Work out the finished part from the listing and answer in its coordinate system (mm). A direction names the side the tool comes from. Round coordinates to 2 decimals unless told otherwise and drop trailing zeros. Loops run counter-clockwise (first coordinate to the right, second up) from the corner with the lowest first, then second, coordinate; pieces in that order, holes last.
```python
from build123d import *

# Parameters (mm, degrees)
F0_W         = 279.4
F0_H         = 482.6
F1_DEPTH     = 25.4
F2_R         = 5.08
F3_R         = 5.08
F4_W         = 176.9686788321
F4_H         = 19.3408131599
F5_DEPTH     = 25.4
F6_W         = 167.2982573509
F6_H         = 19.3408429623
F7_DEPTH     = 25.4
F8_W         = 152.4
F8_H         = 152.4
F9_DEPTH     = 25.4
F10_T        = 2.54
F10_T3_DEPTH = 157.48
F10_T5_DEPTH = 157.48
F10_T7_DEPTH = 30.48
F11_W        = 39.6487191319
F11_H        = 63.5
F12_DEPTH    = 25.4
F13_R        = 7.7119354401
F14_DEPTH    = 50.8


# Not quite as in the source:
# - a shell that OpenCascade refuses in one call is made with other operations: the cavity is built on its own and cut out


with BuildPart() as f1:
    # F0 (on Right) → F1 (new body)
    with BuildSketch(Plane.YZ):
        Rectangle(F0_W, F0_H)
    extrude(amount=F1_DEPTH)

    # F2
    f2_edges = [f1.edges().sort_by_distance(p)[0] for p in [
        (0, 139.7, 0),
        (0, 0, 241.3),
        (0, -139.7, 0),
        (0, 0, -241.3),
    ]]
    fillet(f2_edges, radius=F2_R)

    # F3
    f3_edges = [f1.edges().sort_by_distance(p)[0] for p in [
        (25.4, 139.7, 0),
        (25.4, 0, 241.3),
        (25.4, -139.7, 0),
        (25.4, 0, -241.3),
    ]]
    fillet(f3_edges, radius=F3_R)

    # F4 (on face) → F5 (cut)
    with BuildSketch(Plane(origin=(0, 0, 0), x_dir=(0, -1, 0), z_dir=(-1, 0, 0))):
        with Locations((0, 155.2102416754)):
            Rectangle(F4_W, F4_H)
    extrude(amount=-F5_DEPTH, mode=Mode.SUBTRACT)

    # F6 (on face) → F7 (cut)
    with BuildSketch(Plane.YZ.offset(25.4)):
        with Locations((0, 109.7592636943)):
            Rectangle(F6_W, F6_H)
    extrude(amount=-F7_DEPTH, mode=Mode.SUBTRACT)

    # F8 (on face) → F9 (join)
    with BuildSketch(Plane(origin=(0, 0, 0), x_dir=(0, -1, 0), z_dir=(-1, 0, 0))):
        Rectangle(F8_W, F8_H)
    extrude(amount=F9_DEPTH)

    # F10: shell of thickness 2.54, made by hand


with BuildPart() as f10_core1:
    # F10_t2: copy of F1
    add(f1.part)

    # the walls: a layer under each face that stays
    f10_faces = [f10_core1.faces().sort_by_distance(p)[0] for p in [
        (12.7, 139.7, 0),
        (12.7, 0, -241.3),
        (23.912103095, 138.2121018019, 0),
        (1.4878975516, 138.2121024484, 0),
        (12.7, 0, 241.3),
        (12.7, -139.7, 0),
        (23.912103095, 0, -239.8121018019),
        (1.4878975516, 0, -239.8121024484),
        (25.4, 0, 0),
        (23.912103095, 0, 239.8121018019),
        (0, -89.7466666667, -157.48),
        (1.4878975516, 0, 239.8121024484),
        (23.912103095, -138.2121018019, 0),
        (1.4878975516, -138.2121024484, 0),
        (12.7, 0, 119.4296851754),
        (12.7, -83.6491286755, 109.7592636943),
        (12.7, 0, 100.0888422132),
        (12.7, 83.6491286755, 109.7592636943),
        (12.7, -88.484339416, 155.2102416754),
        (12.7, 0, 145.5398350954),
        (12.7, 0, 164.8806482553),
        (12.7, 88.484339416, 155.2102416754),
        (-12.7, -76.2, 0),
        (-12.7, 0, -76.2),
        (-12.7, 76.2, 0),
        (-12.7, 0, 76.2),
    ]]
    thicken(f10_faces, amount=-F10_T, mode=Mode.SUBTRACT)

    # F10_s4 → F10_t3 (cut)
    with BuildSketch(Plane.XY.offset(-78.74)):
        Polygon((-0.0254, -76.2254), (2.54, -76.2), (2.54, -73.66), (0, -73.66), align=None)
        Polygon((-0.0254, 76.2254), (2.54, 76.2), (2.54, 73.66), (0, 73.66), align=None)
    extrude(amount=F10_T3_DEPTH, mode=Mode.SUBTRACT)

    # F10_s6 → F10_t5 (cut)
    with BuildSketch(Plane.XZ.offset(-78.74)):
        Polygon((-0.0254, -76.2254), (2.54, -76.2), (2.54, -73.66), (0, -73.66), align=None)
        Polygon((-0.0254, 76.2254), (2.54, 76.2), (2.54, 73.66), (0, 73.66), align=None)
    extrude(amount=F10_T5_DEPTH, mode=Mode.SUBTRACT)

    # F10_s8 → F10_t7 (cut)
    with BuildSketch(Plane.YZ.offset(-2.54)):
        Polygon((83.6237286755, 119.4042851754), (83.6491286755, 121.9696851754), (86.1891286755, 121.9696851754), (86.1891286755, 119.4296851754), align=None)
        Polygon((-83.6237286755, 119.4042851754), (-83.6491286755, 121.9696851754), (-86.1891286755, 121.9696851754), (-86.1891286755, 119.4296851754), align=None)
        Polygon((-83.6237286755, 100.1142422132), (-86.1891286755, 100.0888422132), (-86.1891286755, 97.5488422132), (-83.6491286755, 97.5488422132), align=None)
        Polygon((83.6237286755, 100.1142422132), (83.6491286755, 97.5488422132), (86.1891286755, 97.5488422132), (86.1891286755, 100.0888422132), align=None)
        Polygon((-88.458939416, 145.5652350954), (-91.024339416, 145.5398350954), (-91.024339416, 142.9998350954), (-88.484339416, 142.9998350954), align=None)
        Polygon((-88.458939416, 164.8552482553), (-91.024339416, 164.8806482553), (-91.024339416, 167.4206482553), (-88.484339416, 167.4206482553), align=None)
        Polygon((88.458939416, 145.5652350954), (88.484339416, 142.9998350954), (91.024339416, 142.9998350954), (91.024339416, 145.5398350954), align=None)
        Polygon((88.458939416, 164.8552482553), (88.484339416, 167.4206482553), (91.024339416, 167.4206482553), (91.024339416, 164.8806482553), align=None)
    extrude(amount=F10_T7_DEPTH, mode=Mode.SUBTRACT)


with BuildPart() as f1_1:
    add(f1.part)

    # what is left inside the walls is the cavity
    f10_cavity = [f10_core1.part.solids().sort_by_distance(p)[0] for p in [
        (22.8346, 0, -78.74),
    ]]
    add(f10_cavity, mode=Mode.SUBTRACT)

    # F11 (on face) → F12 (join)
    with BuildSketch(Plane(origin=(0, 0, 0), x_dir=(0, -1, 0), z_dir=(-1, 0, 0))):
        with Locations((0, 44.45)):
            Rectangle(F11_W, F11_H)
    extrude(amount=F12_DEPTH)

    # F13 (on face) → F14 (cut)
    with BuildSketch(Plane(origin=(0, 19.824359566, 0), x_dir=(-1, 0, 0), z_dir=(0, 1, 0))):
        with Locations((12.3025374487, 43.18)):
            Circle(F13_R)
    extrude(amount=-F14_DEPTH, mode=Mode.SUBTRACT)


solid = f1_1.part
```
1. Find section D-D (z = -185.5). Write down the section's boundary in (x, y), then the cut area to 3 significant figures.
Answer key:
outline: (0, -134.62) arc R5.08 ccw to (5.08, -139.7) - (20.32, -139.7) arc R5.08 ccw to (25.4, -134.62) - (25.4, 134.62) arc R5.08 ccw to (20.32, 139.7) - (5.08, 139.7) arc R5.08 ccw to (0, 134.62) - close; hole (2.54, -134.62) arc R2.54 ccw to (5.08, -137.16) - (20.32, -137.16) arc R2.54 ccw to (22.86, -134.62) - (22.86, 134.62) arc R2.54 ccw to (20.32, 137.16) - (5.08, 137.16) arc R2.54 ccw to (2.54, 134.62) - close
area: 1,510 mm2
2. Consider probe 1 along X at (y, z) = (9, 43); probe 2 along Z at (x, y) = (13, -1.5); probe 3 along Y at (x, z) = (-9, 37). Determine where each line is inside the solid, lowest interval first.
Answer key:
probe 1: x = -25.4 to -20.01, -4.59 to 0, 22.86 to 25.4
probe 2: z = -241.3 to -238.76, 97.55 to 100.09, 119.43 to 121.97, 143 to 145.54, 164.88 to 167.42, 238.76 to 241.3
probe 3: y = -76.2 to -73.66, 73.66 to 76.2
3. Find section C-C (z = 43.18). Give the number of separate pieces and of enclosed holes in the cut face, then the cut area to 3 significant figures.
Answer key:
separate pieces: 3
enclosed holes: 0
area: 1,660 mm2
4. Given pin 1 (3 mm diameter, centred on x = 0.5, z = -131.5, fed in from +Y); pin 2 (10 mm diameter, centred on x = -9.5, y = -18.5, fed in from +Z); pin 3 (4 mm diameter, centred on x = -19, z = 13.5, fed in from -Y), each flat-ended and moving along its own axis, determine where each tip first touches the part or whether it passes through.
Answer key:
pin 1: stops at y = 138.66
pin 2: stops at z = 76.2
pin 3: stops at y = -76.2
5. Which of the six approach directions +Z, -Z, +X, -X, +Y, -Y give full straight-line access (tool end or side, diameter ignored) to faces 4 (the face through (-21, -19.824, 43)), 5 (the face through (13, 1, 164.881)), 6 (the face through (13, 139.7, -3)), 7 (the face through (13, -1, 167.421)), 8 (the face through (25.4, -2, 3))?
Answer key:
face 4: -X
face 5: +X, -X
face 6: +Z, -Z, +X, -X, +Y
face 7: none
face 8: +Z, -Z, +X, +Y, -Y
6. Find section B-B (y = -104.5). Write down the section's boundary in (x, z).
Answer key:
outline: (0, -236.22) arc R5.08 ccw to (5.08, -241.3) - (20.32, -241.3) arc R5.08 ccw to (25.4, -236.22) - (25.4, 236.22) arc R5.08 ccw to (20.32, 241.3) - (5.08, 241.3) arc R5.08 ccw to (0, 236.22) - close; hole (2.54, -236.22) arc R2.54 ccw to (5.08, -238.76) - (20.32, -238.76) arc R2.54 ccw to (22.86, -236.22) - (22.86, 236.22) arc R2.54 ccw to (20.32, 238.76) - (5.08, 238.76) arc R2.54 ccw to (2.54, 236.22) - close
7. Determine the mould class of faces 1 (the face through (13, 1, 145.54)), 2 (the face through (-25.4, 17, 46)), 3 (the face through (-13, 1, -76.2)) for opening direction Z: +Z half, -Z half, draft (parallel to the pull), parting line (faces both ways), or undercut.
Answer key:
face 1: undercut
face 2: draft
face 3: -Z half
8. Find section A-A (x = -13.5). Write down the section's boundary in (y, z).
Answer key:
outline: (-76.2, -76.2) - (76.2, -76.2) - (76.2, 76.2) - (-76.2, 76.2) - close; (-19.82, 12.7) - (19.82, 12.7) - (19.82, 35.56) - (-19.82, 35.56) - close; hole (-73.66, -73.66) - (73.66, -73.66) - (73.66, 73.66) - (19.82, 73.66) - (19.82, 50.8) - (-19.82, 50.8) - (-19.82, 73.66) - (-73.66, 73.66) - close
